```python
from build123d import *

# Parameters (mm, degrees)
BOSS_EXTRUDE1_DEPTH = 25.4
CUT_EXTRUDE1_DEPTH  = 25.4
CUT_EXTRUDE2_REACH  = 158.576
CUT_EXTRUDE6_REACH  = 161.131
CUT_EXTRUDE7_REACH  = 161.131
SKETCH8_R           = 2.159
SKETCH8_W           = 42.6085
SKETCH8_H           = 20.32
FILLET2_R           = 6.35
FILLET1_R           = 1.5875


with BuildPart() as part:
    # Sketch1 → Boss-Extrude1 (new body)
    with BuildSketch(Plane(origin=(0, 0, 0), x_dir=(1, 0, 0), z_dir=(0, 1, 0))):
        with BuildLine():
            Line((152.4, -25.4), (83.304393675, -25.4))
            Line((83.304393675, -25.4), (77.805132361, -15.875))
            Line((77.805132361, -15.875), (70.472783942, -3.175))
            ThreePointArc((70.472783942, -3.175), (63.5, 3.797783942), (53.975, 6.35))
            Line((53.975, 6.35), (0, 6.35))
            Line((0, 6.35), (0, -6.35))
            Line((0, -6.35), (53.975, -6.35))
            ThreePointArc((53.975, -6.35), (57.15, -7.200738686), (59.474261314, -9.525))
            Line((59.474261314, -9.525), (66.806609733, -22.225))
            ThreePointArc((66.806609733, -22.225), (73.779393675, -29.197783942), (83.304393675, -31.75))
            Line((83.304393675, -31.75), (152.4, -31.75))
            Line((152.4, -31.75), (152.4, -25.4))
        make_face()
    extrude(amount=BOSS_EXTRUDE1_DEPTH)

    # Sketch3 → Cut-Extrude1 (cut)
    with BuildSketch(Plane.XY.offset(6.35)):
        with BuildLine():
            ThreePointArc((7.08025, 9.609467329), (8.164970659, 8.164970659), (9.609467329, 7.08025))
            Line((9.609467329, 7.08025), (15.790532671, 7.08025))
            ThreePointArc((15.790532671, 7.08025), (17.235029341, 8.164970659), (18.31975, 9.609467329))
            Line((18.31975, 9.609467329), (18.31975, 15.790532671))
            ThreePointArc((18.31975, 15.790532671), (17.235029341, 17.235029341), (15.790532671, 18.31975))
            Line((15.790532671, 18.31975), (9.609467329, 18.31975))
            ThreePointArc((9.609467329, 18.31975), (8.164970659, 17.235029341), (7.08025, 15.790532671))
            Line((7.08025, 15.790532671), (7.08025, 9.609467329))
        make_face()
    extrude(amount=-CUT_EXTRUDE1_DEPTH, mode=Mode.SUBTRACT)

    # Sketch4 → Cut-Extrude2 (cut, up to next)
    with BuildSketch(Plane.XY.offset(6.35), mode=Mode.PRIVATE) as cut_extrude2_sk1:
        with BuildLine():
            Line((0, 12.7), (0, 0))
            Line((0, 0), (12.7, 0))
            ThreePointArc((12.7, 0), (3.719743879, 3.719743879), (0, 12.7))
        make_face()
    cut_extrude2_tool1 = extrude(cut_extrude2_sk1.sketch, amount=-CUT_EXTRUDE2_REACH, mode=Mode.PRIVATE) & part.part
    # Sketch4 → Cut-Extrude2 (cut, up to next)
    with BuildSketch(Plane.XY.offset(6.35), mode=Mode.PRIVATE) as cut_extrude2_sk2:
        with BuildLine():
            Line((0, 25.4), (0, 12.7))
            ThreePointArc((0, 12.7), (3.719743879, 21.680256121), (12.7, 25.4))
            Line((12.7, 25.4), (0, 25.4))
        make_face()
    cut_extrude2_tool2 = extrude(cut_extrude2_sk2.sketch, amount=-CUT_EXTRUDE2_REACH, mode=Mode.PRIVATE) & part.part
    add(cut_extrude2_tool1.solids().sort_by_distance((2.836773, 2.836773, 6.35))[0], mode=Mode.SUBTRACT)
    add(cut_extrude2_tool2.solids().sort_by_distance((2.836773, 22.563227, 6.35))[0], mode=Mode.SUBTRACT)

    # Sketch7 → Cut-Extrude6 (cut, up to next)
    with BuildSketch(Plane.XY.offset(31.75), mode=Mode.PRIVATE) as cut_extrude6_sk1:
        with BuildLine():
            ThreePointArc((139.7, 25.4), (148.680256121, 21.680256121), (152.4, 12.7))
            Line((152.4, 12.7), (152.4, 25.4))
            Line((152.4, 25.4), (139.7, 25.4))
        make_face()
    cut_extrude6_tool1 = extrude(cut_extrude6_sk1.sketch, amount=-CUT_EXTRUDE6_REACH, mode=Mode.PRIVATE) & part.part
    # Sketch7 → Cut-Extrude6 (cut, up to next)
    with BuildSketch(Plane.XY.offset(31.75), mode=Mode.PRIVATE) as cut_extrude6_sk2:
        with BuildLine():
            ThreePointArc((152.4, 12.7), (148.680256121, 3.719743879), (139.7, 0))
            Line((139.7, 0), (152.4, 0))
            Line((152.4, 0), (152.4, 12.7))
        make_face()
    cut_extrude6_tool2 = extrude(cut_extrude6_sk2.sketch, amount=-CUT_EXTRUDE6_REACH, mode=Mode.PRIVATE) & part.part
    add(cut_extrude6_tool1.solids().sort_by_distance((149.563227, 22.563227, 31.75))[0], mode=Mode.SUBTRACT)
    add(cut_extrude6_tool2.solids().sort_by_distance((149.563227, 2.836773, 31.75))[0], mode=Mode.SUBTRACT)

    # Sketch8 → Cut-Extrude7 (cut, up to next)
    with BuildSketch(Plane.XY.offset(31.75), mode=Mode.PRIVATE) as cut_extrude7_sk1:
        with Locations((138.811, 7.8486)):
            Circle(SKETCH8_R)
    cut_extrude7_tool1 = extrude(cut_extrude7_sk1.sketch, amount=-CUT_EXTRUDE7_REACH, mode=Mode.PRIVATE) & part.part
    # Sketch8 → Cut-Extrude7 (cut, up to next)
    with BuildSketch(Plane.XY.offset(31.75), mode=Mode.PRIVATE) as cut_extrude7_sk2:
        with Locations(Location((138.811, 17.5514, 0), (0, 0, 180))):
            Circle(SKETCH8_R)
    cut_extrude7_tool2 = extrude(cut_extrude7_sk2.sketch, amount=-CUT_EXTRUDE7_REACH, mode=Mode.PRIVATE) & part.part
    # Sketch8 → Cut-Extrude7 (cut, up to next)
    with BuildSketch(Plane.XY.offset(31.75), mode=Mode.PRIVATE) as cut_extrude7_sk3:
        with Locations(Location((89.789, 7.8486, 0), (0, 0, 180))):
            Circle(SKETCH8_R)
    cut_extrude7_tool3 = extrude(cut_extrude7_sk3.sketch, amount=-CUT_EXTRUDE7_REACH, mode=Mode.PRIVATE) & part.part
    # Sketch8 → Cut-Extrude7 (cut, up to next)
    with BuildSketch(Plane.XY.offset(31.75), mode=Mode.PRIVATE) as cut_extrude7_sk4:
        with Locations((89.789, 17.5514)):
            Circle(SKETCH8_R)
    cut_extrude7_tool4 = extrude(cut_extrude7_sk4.sketch, amount=-CUT_EXTRUDE7_REACH, mode=Mode.PRIVATE) & part.part
    # Sketch8 → Cut-Extrude7 (cut, up to next)
    with BuildSketch(Plane.XY.offset(31.75), mode=Mode.PRIVATE) as cut_extrude7_sk5:
        with Locations((114.3, 12.7)):
            Rectangle(SKETCH8_W, SKETCH8_H)
    cut_extrude7_tool5 = extrude(cut_extrude7_sk5.sketch, amount=-CUT_EXTRUDE7_REACH, mode=Mode.PRIVATE) & part.part
    add(cut_extrude7_tool1.solids().sort_by_distance((138.811, 7.8486, 31.75))[0], mode=Mode.SUBTRACT)
    add(cut_extrude7_tool2.solids().sort_by_distance((138.811, 17.5514, 31.75))[0], mode=Mode.SUBTRACT)
    add(cut_extrude7_tool3.solids().sort_by_distance((89.789, 7.8486, 31.75))[0], mode=Mode.SUBTRACT)
    add(cut_extrude7_tool4.solids().sort_by_distance((89.789, 17.5514, 31.75))[0], mode=Mode.SUBTRACT)
    add(cut_extrude7_tool5.solids().sort_by_distance((114.3, 12.7, 31.75))[0], mode=Mode.SUBTRACT)

    # Fillet2
    fillet2_edges = [part.edges().sort_by_distance(p)[0] for p in [
        (83.304393675, 12.7, 25.4),
    ]]
    fillet(fillet2_edges, radius=FILLET2_R)

    # Fillet1
    fillet1_edges = [part.edges().sort_by_distance(p)[0] for p in [
        (75.972045256, 0, 12.7),
        (111.502196837, 0, 31.75),
        (113.335283942, 25.4, 25.4),
        (113.335283942, 0, 25.4),
        (83.795567884, 0, 24.549261314),
        (83.795567884, 25.4, 24.549261314),
        (73.779393675, 0, 29.197783942),
        (63.140435523, 0, 15.875),
        (57.15, 0, 7.200738686),
        (63.5, 0, -3.797783942),
        (57.15, 25.4, 7.200738686),
        (63.140435523, 25.4, 15.875),
        (73.779393675, 25.4, 29.197783942),
        (111.502196837, 25.4, 31.75),
        (75.972045256, 25.4, 12.7),
        (63.5, 25.4, -3.797783942),
        (33.3375, 25.4, -6.35),
        (33.3375, 25.4, 6.35),
        (0, 12.7, 6.35),
        (0, 12.7, -6.35),
        (33.3375, 0, 6.35),
        (33.3375, 0, -6.35),
        (152.4, 12.7, 31.75),
        (152.4, 12.7, 25.4),
    ]]
    fillet(fillet1_edges, radius=FILLET1_R)


solid = part.part
```
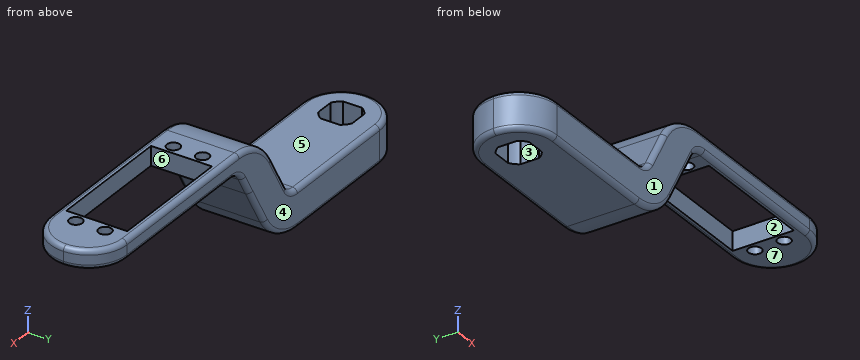
CAD build for the part. Positions are in the model's coordinates, mm. Face numbers are marked on the shaded views. A direction names the side the tool comes from. Round coordinates to 2 decimals unless told otherwise and drop trailing zeros. One line per question, with ' | ' between items.
1. Mould opens along Y. For the marked faces 1, 2, 3 and 4 say: pulls with the +Y half, pulls with the -Y half, needs draft (parallel to the pull), parting line crosses it, or undercut.
Working result:
face 1: pulls with the -Y half | face 2: undercut | face 3: undercut | face 4: pulls with the +Y half
2. Pin check, flat tips, straight feed: pin 1 Ø12 at (y, z) = (12, 2) entering from -X; pin 2 Ø7 at (y, z) = (9, 28) entering from +X; pin 3 Ø5 at (x, y) = (90.5, 19) entering from -Z; pin 4 Ø3 at (y, z) = (12.5, 3) entering from +X. Stop position of each tip, or through.
Working result:
pin 1: x = 0 | pin 2: x = 152.4 | pin 3: z = 25.4 | pin 4: x = 71.24
3. Cut at C-C on z = 28.5. Count the separate pieces of the cut face and the enclosed holes in it, and give its area (3 significant figures).
Working result:
separate pieces: 1 | enclosed holes: 5 | area: 1,030 mm2
4. Which spindle directions (+Z, -Z, +X, -X, +Y, -Y) get a long thin tool onto all of the face, cutting with end or side? Do the marked faces 5, 6 and 7. Say none if no direction does.
Working result:
face 5: +Z, -X, +Y, -Y | face 6: +Z, -Z | face 7: -Z, +X, +Y, -Y
5. Probe L1, parallel to Y at x = 124, z = 30; L2, parallel to Z at x = 37, y = 5; L3, parallel to Z at x = 119, y = 2. List the from-to ranges inside material, lowest first. Write a range as from..to.
Working result:
L1: 0..2.54, 22.86..25.4 | L2: -6.35..6.35 | L3: 25.4..31.75
